```python
from build123d import *

# Parameters (mm, degrees)
SKETCH_1_R      = 1.5
EXTRUDE_1_DEPTH = 1.6
FILLET_1_R      = 1.5


with BuildPart() as part:
    # 草图1 → 凸台-拉伸1 (new body)
    with BuildSketch(Plane.XY):
        Polygon((0, 0), (28.5, 0), (28.5, 29.5), (2.5, 29.5), (0, 29.5), align=None)
        with Locations((2.5, 27)):
            Circle(SKETCH_1_R, mode=Mode.SUBTRACT)
        with Locations((26, 27)):
            Circle(SKETCH_1_R, mode=Mode.SUBTRACT)
        with Locations((26, 2.5)):
            Circle(SKETCH_1_R, mode=Mode.SUBTRACT)
        with Locations((2.5, 2.5)):
            Circle(SKETCH_1_R, mode=Mode.SUBTRACT)
    extrude(amount=EXTRUDE_1_DEPTH)

    # 圆角1
    fillet_1_edges = [part.edges().sort_by_distance(p)[0] for p in [
        (0, 29.5, 0.8),
        (28.5, 29.5, 0.8),
        (28.5, 0, 0.8),
        (0, 0, 0.8),
    ]]
    fillet(fillet_1_edges, radius=FILLET_1_R)


solid = part.part
```
Check sheet for the modelled part. Datum: model origin and axes. Units: mm. Coordinates: 2 decimals unless noted, no trailing zeros. Write each loop counter-clockwise with the first axis right and the second up, starting at its lowest first coordinate (ties: lowest second). Pieces come first, ordered by that corner, then holes. Notation, with made-up numbers: (-35, 0) -> (-11, 0) arc R22 ccw to (-11, 38) -> close; hole circle Ø1 at (35, -4.75). An arc over 180 degrees is marked (long way). Use a Markdown table: item, result.
1. Go/stop test with a flat-tipped pin: pin 1 Ø1.8 at (x, y) = (26, 2.5) entering from +Z. Record where the tip stops, or that it passes through.
Reported:
| item | result |
|---|---|
| pin 1 | passes through |
2. Sectioned sample at B-B (y = 2.5). Enter the section's corners in (x, z), plus the area to 3 significant figures.
Reported:
| item | result |
|---|---|
| outline | (0, 0) -> (1, 0) -> (1, 1.6) -> (0, 1.6) -> close; (4, 0) -> (24.5, 0) -> (24.5, 1.6) -> (4, 1.6) -> close; (27.5, 0) -> (28.5, 0) -> (28.5, 1.6) -> (27.5, 1.6) -> close |
| area | 36.0 mm2 |
3. Release check for a two-part mould opening along X. For faces 1 (the cylindrical face through (25.805, 28.487, 0.789)), 2 (the flat face through (14, 29.5, 1)), 3 (the cylindrical face through (2.175, 1.036, 0.789)), 4 (the cylindrical face through (0.45, 0.43, 0.81)) record: pulls with the +X half, pulls with the -X half, needs draft (parallel to the pull), parting line crosses it, or undercut.
Reported:
| item | result |
|---|---|
| face 1 | undercut |
| face 2 | needs draft |
| face 3 | undercut |
| face 4 | pulls with the -X half |
4. Scan lines: line 1 along Y through (x, z) = (26, 0.2); line 2 along X through (y, z) = (26, 1.15); line 3 along X through (y, z) = (3.75, 0.45). Record each from-to range of solid material in increasing order.
Reported:
| item | result |
|---|---|
| line 1 | y = 0 to 1, 4 to 25.5, 28.5 to 29.5 |
| line 2 | x = 0 to 1.38, 3.62 to 24.88, 27.12 to 28.5 |
| line 3 | x = 0 to 1.67, 3.33 to 25.17, 26.83 to 28.5 |
5. Sectioned sample at C-C (z = 0.75). Enter the section's corners in (x, y), plus the area to 3 significant figures.
Reported:
| item | result |
|---|---|
| outline | (0, 1.5) arc R1.5 ccw to (1.5, 0) -> (27, 0) arc R1.5 ccw to (28.5, 1.5) -> (28.5, 28) arc R1.5 ccw to (27, 29.5) -> (1.5, 29.5) arc R1.5 ccw to (0, 28) -> close; hole circle Ø3 at (2.5, 2.5); hole circle Ø3 at (2.5, 27); hole circle Ø3 at (26, 2.5); hole circle Ø3 at (26, 27) |
| area | 811 mm2 |
6. Sectioned sample at A-A (x = 26). Enter the section's corners in (y, z), plus the area to 3 significant figures.
Reported:
| item | result |
|---|---|
| outline | (0, 0) -> (1, 0) -> (1, 1.6) -> (0, 1.6) -> close; (4, 0) -> (25.5, 0) -> (25.5, 1.6) -> (4, 1.6) -> close; (28.5, 0) -> (29.5, 0) -> (29.5, 1.6) -> (28.5, 1.6) -> close |
| area | 37.6 mm2 |
